from build123d import *

# Parameters (mm, degrees)
ESQUISSE2_R                  = 11.836112132
BOSS_EXTRU_1_DEPTH           = 4
BOSS_EXTRU_2_START           = -4
BOSS_EXTRU_2_DEPTH           = 4
R_P_TITION_CIRCULAIRE1_COUNT = 11
ESQUISSE6_R                  = 16.559612132
ESQUISSE6_R_2                = 16.059612132
ENL_V_MAT_EXTRU_3_DEPTH      = 24.640803164
CUT_EXTRUDE1_DEPTH           = 10


with BuildPart() as part:
    # Esquisse2 → Boss.-Extru.1 (new body)
    with BuildSketch(Plane.XY):
        Circle(ESQUISSE2_R)
    extrude(amount=BOSS_EXTRU_1_DEPTH)

    # Esquisse3 → Boss.-Extru.2 (add)
    with BuildSketch(Plane.XY.offset(4).offset(BOSS_EXTRU_2_START)):
        with BuildLine():
            Line((-5.344448394, 13.436688428), (-5.305069319, 13.002458629))
            ThreePointArc((-5.305069319, 13.002458629), (-5.28156066, 12.313590322), (-5.335640108, 11.626445786))
            ThreePointArc((-5.335640108, 11.626445786), (-5.684064042, 10.675034327), (-6.399085338, 9.957171146))
            ThreePointArc((-6.399085338, 9.957171146), (-3.334618134, 11.356666425), (0, 11.836112132))
            ThreePointArc((0, 11.836112132), (-0.989620329, 12.053447371), (-1.797105063, 12.665453421))
            ThreePointArc((-1.797105063, 12.665453421), (-2.214097973, 13.214278633), (-2.566751555, 13.806501271))
            Line((-2.566751555, 13.806501271), (-2.768386123, 14.193088558))
            ThreePointArc((-2.768386123, 14.193088558), (-3.562335584, 15.213850424), (-4.665381866, 15.888831486))
            ThreePointArc((-4.665381866, 15.888831486), (-5.228401135, 14.72464944), (-5.344448394, 13.436688428))
        make_face()
    boss_extru_2 = extrude(amount=BOSS_EXTRU_2_DEPTH)

    # Répétition circulaire1: Boss.-Extru.2 ×11 about axis
    r_p_tition_circulaire1_axis = Axis((0, 0, 0), (0, 0, 1))
    for i in range(1, R_P_TITION_CIRCULAIRE1_COUNT):
        add(boss_extru_2.rotate(r_p_tition_circulaire1_axis, i * 360 / R_P_TITION_CIRCULAIRE1_COUNT))

    # Esquisse6 → Enlèv. mat.-Extru.3 (cut, through all)
    with BuildSketch(Plane(origin=(0, 0, 0), x_dir=(-1, 0, 0), z_dir=(0, 0, -1))):
        Circle(ESQUISSE6_R)
        Circle(ESQUISSE6_R_2, mode=Mode.SUBTRACT)
    extrude(amount=-ENL_V_MAT_EXTRU_3_DEPTH, mode=Mode.SUBTRACT)

    # Sketch1 → Cut-Extrude1 (cut)
    with BuildSketch(Plane.XY.offset(4)):
        with BuildLine():
            Line((-5.02, 3.39), (-5.02, -3.39))
            ThreePointArc((-5.02, -3.39), (0, -6.05743345), (5.02, -3.39))
            Line((5.02, -3.39), (5.02, 3.39))
            ThreePointArc((5.02, 3.39), (0, 6.05743345), (-5.02, 3.39))
        make_face()
    extrude(amount=-CUT_EXTRUDE1_DEPTH, mode=Mode.SUBTRACT)


solid = part.part
Source: CAD feature listing. Evaluate the final solid. Frame: model axes, mm. A direction names the side the tool comes from. Coordinates: 2 decimals unless noted, no trailing zeros. Loops run counter-clockwise (first coordinate to the right, second up) from the corner with the lowest first, then second, coordinate; pieces in that order, holes last. Notation, with made-up numbers: (49, 8) - (60, 8) arc R22 cw to (60, 30) - close; hole circle Ø5 at (29.5, 70.25). An arc over 180 degrees is marked (long way). Return JSON: item names as keys, results as strings.
Q1. Section A-A, the plane x = 4.5. Return loops of the section in (y, z).
Results:
{"outline": "(-11.31, 0) - (-4.05, 0) - (-4.05, 4) - (-11.31, 4) - close; (4.05, 0) - (15.42, 0) - (15.42, 4) - (4.05, 4) - close"}
Q2. Access query for faces 1 (the cylindrical face through (-11.1, 7.5, 2)), 2 (the cylindrical face through (7.367, -13.411, 1.972)), 3 (the cylindrical face through (-0.083, -6.057, 2.028)), 4 (the cylindrical face through (12.772, -4.079, 1.972)). Directions: +Z, -Z, +X, -X, +Y, -Y. A direction counts if a zero-diameter tool reaches every point of the face in a straight line with its end or side. Return the directions, or none.
Results:
{"face 1": "+Z, -Z, -X", "face 2": "+Z, -Z, -Y", "face 3": "+Z, -Z", "face 4": "+Z, -Z, +X"}
Q3. Material intervals for line 1 along X through (y, z) = (-13, 2.7); line 2 along X through (y, z) = (-2, 1.65); line 3 along Y through (x, z) = (12, 0.2), sorted ascending.
Results:
{"line 1": "-9.15 to -6.82, -1.7 to 1.7, 6.82 to 9.15", "line 2": "-11.69 to -5.02, 5.02 to 11.69", "line 3": "-7.08 to -3.19, -0.85 to 3.72, 8.76 to 10.67"}
Q4. Contact query for flat-ended pins moving along their axis: P1, Ø1.5, axis at x = 8.5, z = 0.5, coming from the +Y side; P2, Ø1, axis at y = 3.5, z = 3, coming from the -X side. Output: stop coordinate, or through.
Results:
{"P1": "y = 10.03", "P2": "x = -15.49"}
Q5. Section B-B, the plane x = -7.5. Return loops of the section in (y, z).
Results:
{"outline": "(-13.49, 0) - (9.59, 0) - (9.59, 4) - (-13.49, 4) - close"}
Q6. Mould query, pull axis X, two halves, no side actions, for faces 5 (the cylindrical face through (15, 3.2, 2)), 6 (the cylindrical face through (-15, 3.2, 2)), 7 (the cylindrical face through (-13.47, -7.3, 1.97)). Classes: released by +X, released by -X, zero draft, split by the parting line, or undercut.
Results:
{"face 5": "released by +X", "face 6": "released by -X", "face 7": "undercut"}
